For this review, take the finished solid that the model builds, in its own axes (mm). A direction names the side the tool comes from. Give positions to 0.01 mm unless a question says otherwise; leave off trailing zeros. Order: outer loops, then holes, each group sorted by start corner. A loop starts at its lowest first (then second) coordinate and runs counter-clockwise, first axis right, second up. Notation, with made-up numbers: (32.25, 88.5) -> (36.25, 88.5) arc R29 cw to (36.25, 117.5) -> close; hole circle Ø8 at (20, -4.75). An arc over 180 degrees is marked (long way). Return JSON: item names as keys, results as strings. Group by question number.
1) Add section D-D (z = 11.5). Give the boundary of the cut face in (x, y).
2) The part is to be moulded in two halves that separate along Y. For faces 1 (the face through (-6.35, 125, 1)), 2 (the face through (-206, 129, 50.8)), 3 (the face through (-200.355, 2.173, 48.509)), say which applies: released by +Y, released by -Y, zero draft, split by the parting line, or undercut.
3) Add section B-B (y = 95). State how many separate pieces and enclosed holes the cut face has, then the cut area to 3 significant figures.
4) Insertion check: P1, Ø12, axis at x = -286, z = 20, coming from the -Y side; P2, Ø6, axis at y = 94.5, z = -60.5, coming from the +X side; P3, Ø12, axis at x = -315, y = 119.5, coming from the +Z side; P4, Ø3, axis at x = -232, y = 212.5, coming from the -Z side. Each pin has a flat end and moves straight along its axis. Give the tip position at first contact, or say it passes through.
5) To check wall thickness, follow line 1 along Y through (x, z) = (-254, 19); line 2 along Z through (x, y) = (-133, 14.5); line 3 along Y through (x, z) = (-37.5, -3.5). State the ranges of each line that lie inside material, in increasing order.
6) Add section A-A (x = -361). Give the boundary of the cut face in (y, z).
7) For faces 4 (the face through (-206, 129, -44.45)), 5 (the face through (-78.176, 84.626, -63.322)), 6 (the face through (-78.176, 84.626, 63.322)), list the 3-axis set-ups (+Z, -Z, +X, -X, +Y, -Y) from which the entire face can be reached by the end or side of a thin tool; tool diameter is ignored.
from build123d import *

# Parameters (mm, degrees)
F0_W     = 406.4
F0_H     = 254
F1_DEPTH = 50.8
F2_R     = 7.62
F3_R     = 38.512752
F4_DEPTH = 50.801
F5_T     = -6.35
F6_R     = 45.404172
F6_R_2   = 38.512752
F7_DEPTH = 25.4


with BuildPart() as f1:
    # F0 (on Top) → F1 (new body)
    with BuildSketch(Plane.XY):
        with Locations((-203.2, 127)):
            Rectangle(F0_W, F0_H)
    extrude(amount=F1_DEPTH)

    # F2
    f2_edges = [f1.edges().sort_by_distance(p)[0] for p in [
        (-406.4, 127, 50.8),
        (-203.2, 0, 50.8),
        (0, 127, 50.8),
        (-203.2, 254, 50.8),
    ]]
    fillet(f2_edges, radius=F2_R)

    # F3 (on face) → F4 (cut, through all)
    with BuildSketch(Plane.XY.offset(50.8)):
        with Locations((-68.333499, 128.950953)):
            Circle(F3_R)
    extrude(amount=-F4_DEPTH, mode=Mode.SUBTRACT)

    # F5
    f5_openings = [f1.faces().sort_by_distance(p)[0] for p in [
        (-209.575826, 126.907769, 0),
    ]]
    offset(amount=F5_T, openings=f5_openings)

    # F6 (on face) → F7 (join)
    with BuildSketch(Plane.XY.offset(50.8)):
        with Locations((-68.333499, 128.950953)):
            Circle(F6_R)
        with Locations((-68.333499, 128.950953)):
            Circle(F6_R_2, mode=Mode.SUBTRACT)
    extrude(amount=F7_DEPTH)

    # F8: F1 across plane


with BuildPart() as f1_1:
    add(f1.part)
    add(f1.part.mirror(Plane.XY))


solid = f1_1.part
Evaluation:
{
 "1": {"outline": "(-406.4, 0) -> (0, 0) -> (0, 254) -> (-406.4, 254) -> close; circle Ø89.73 at (-68.33, 128.95); hole (-400.05, 6.35) -> (-6.35, 6.35) -> (-6.35, 247.65) -> (-400.05, 247.65) -> close; hole circle Ø77.03 at (-68.33, 128.95)"},
 "2": {"face 1": "undercut", "face 2": "zero draft", "face 3": "released by -Y"},
 "3": {"separate pieces": "2", "enclosed holes": "2", "area": "8,980 mm^2"},
 "4": {"P1": "y = 0", "P2": "x = -35.59", "P3": "z = 50.8", "P4": "z = -50.8"},
 "5": {"line 1": "0 to 6.35, 247.65 to 254", "line 2": "-50.8 to -44.45, 44.45 to 50.8", "line 3": "0 to 6.35, 96.36 to 105.87, 152.03 to 161.54, 247.65 to 254"},
 "6": {"outline": "(0, -43.18) arc R7.62 ccw to (7.62, -50.8) -> (246.38, -50.8) arc R7.62 ccw to (254, -43.18) -> (254, 43.18) arc R7.62 ccw to (246.38, 50.8) -> (7.62, 50.8) arc R7.62 ccw to (0, 43.18) -> close; hole (6.35, -43.18) arc R1.27 ccw to (7.62, -44.45) -> (246.38, -44.45) arc R1.27 ccw to (247.65, -43.18) -> (247.65, 43.18) arc R1.27 ccw to (246.38, 44.45) -> (7.62, 44.45) arc R1.27 ccw to (6.35, 43.18) -> close"},
 "7": {"face 4": "none", "face 5": "-Z", "face 6": "+Z"}
}
